The figure shows three views and two pictorial views of one solid part (mm, origin at its lowest corner). Answer the questions. A direction names the side the tool comes from. Coordinates: 2 decimals unless noted, no trailing zeros. Order: outer loops, then holes, each group sorted by start corner. A loop starts at its lowest first (then second) coordinate and runs counter-clockwise, first axis right, second up. Notation, with made-up numbers: M -26,30 L 31,30 A28 ccw 31,49 Z; hole C 20.25,79 d6. An arc over 180 degrees is marked long. Write item = value, one per line. Start each with the question number.
Q1. Determine the mould class of the marked faces 3, 4, 5 and 6 for opening direction Z: released by +Z, released by -Z, zero draft, split by the parting line, or undercut.
Q2. Straight lines are drawn through the part: line 1 along X through (y, z) = (3.5, 8.25) (1 decimal); line 2 along X through (y, z) = (3.5, 5.75); line 3 along Z through (x, y) = (8, 7.5). For each, find the intervals that lie inside material, in ascending order.
Q3. A tool of negligible diameter and unlimited length cuts with its end or side. For the marked faces 1 and 2, from which of +Z, -Z, +X, -X, +Y, -Y can it reach the whole face along a straight path? Write none if from no direction.
Q4. Each of these flat-tipped pins is pushed along its axis until it touches: P1, Ø3, axis at y = 1.5, z = 3, coming from the +X side (1 decimal); P2, Ø2, axis at y = 1.5, z = 3, coming from the +X side. Where does it stop, or does it pass through?
Q5. Find section C-C on y = 7. Give the vertices of the cut face in (x, z).
Q6. Find section B-B on x = 2. Give the vertices of the cut face in (y, z).
Q7. Find section A-A on z = 5. Give the vertices of the cut face in (x, y).
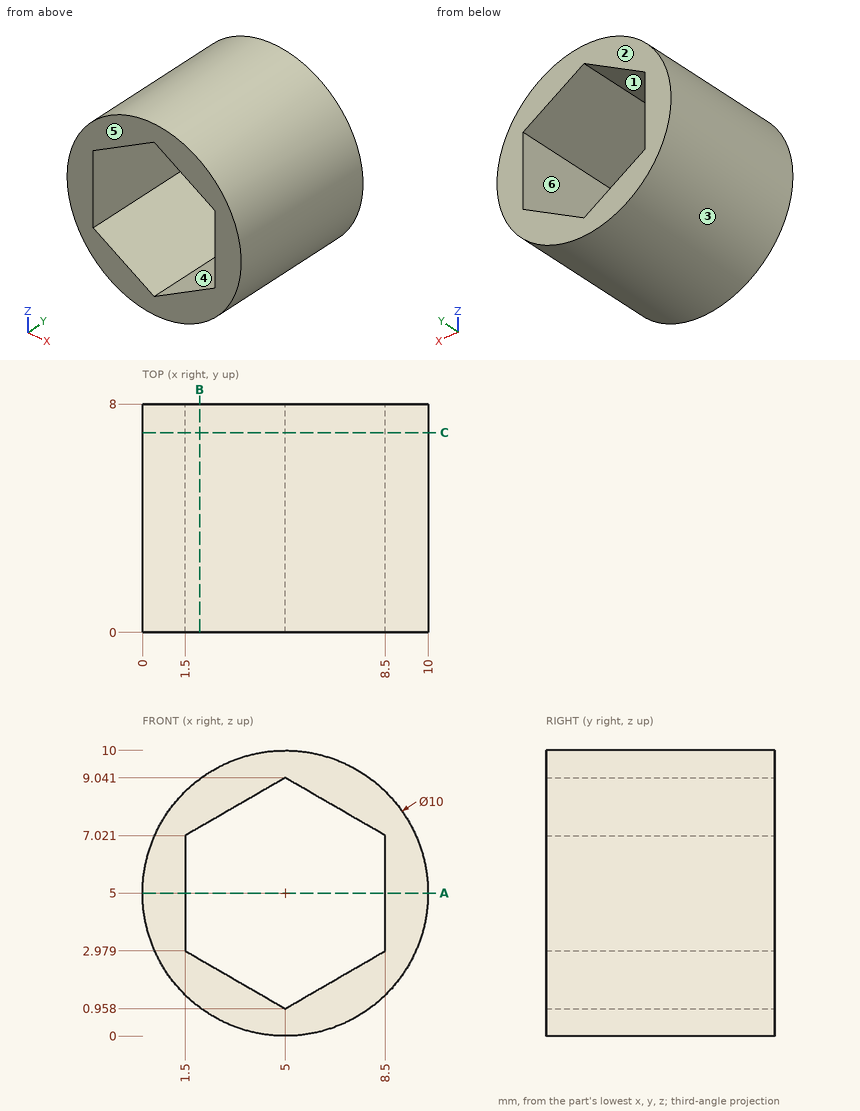
Findings below:
q1.face_3 = split by the parting line
q1.face_4 = undercut
q1.face_5 = zero draft
q1.face_6 = undercut
q2.line_1 = 1.2 to 3.6, 6.4 to 8.8
q2.line_2 = 0.06 to 1.5, 8.5 to 9.94
q2.line_3 = 1 to 2.69, 7.31 to 9
q3.face_1 = +Y, -Y
q3.face_2 = +Z, -Z, +X, -X, +Y
q4.P1 = 10
q4.P2 = 9.9
q5.outline = C 5,5 d10; hole M 1.5,2.98 L 5,0.96 L 8.5,2.98 L 8.5,7.02 L 5,9.04 L 1.5,7.02 Z
q6.outline = M 0,1 L 8,1 L 8,2.69 L 0,2.69 Z; M 0,7.31 L 8,7.31 L 8,9 L 0,9 Z
q7.outline = M 0,0 L 1.5,0 L 1.5,8 L 0,8 Z; M 8.5,0 L 10,0 L 10,8 L 8.5,8 Z
